Work out the finished part from the listing and answer in its coordinate system (mm). A direction names the side the tool comes from. Give positions to 0.01 mm unless a question says otherwise; leave off trailing zeros. Write each loop counter-clockwise with the first axis right and the second up, starting at its lowest first coordinate (ties: lowest second). Pieces come first, ordered by that corner, then holes. Notation, with made-up numbers: (-3, -9) - (35, -9) arc R20 ccw to (35, 23) - close; hole circle Ø10 at (32.25, 83). An arc over 180 degrees is marked (long way). Write item = value, one per line.
from build123d import *

# Parameters (mm, degrees)
SKETCH1_W                   = 190
SKETCH1_H                   = 175
SKETCH1_R                   = 2
SKETCH1_R_2                 = 1.75
BASE_DEPTH                  = 5.4
SKETCH3_R                   = 1.75
LONG_SIDE_CONNECTORS_DEPTH  = 5
SHORT_SIDE_CONNECTORS_DEPTH = 5
MIRROR3_COPY_1_DEPTH        = 5
CUT_EXTRUDE6_START          = -5.4
SKETCH11_R                  = 1.75
CUT_EXTRUDE6_DEPTH          = 179.761105811


with BuildPart() as part:
    # Sketch1 → Base (new body)
    with BuildSketch(Plane(origin=(0, 0, 0), x_dir=(1, 0, 0), z_dir=(0, 1, 0))):
        with Locations((-51.064381671, 5.614281477)):
            Rectangle(SKETCH1_W, SKETCH1_H)
        with Locations(Location((-26.064381671, 30.614281477, 0), (0, 0, 270))):
            Circle(SKETCH1_R, mode=Mode.SUBTRACT)
        with Locations(Location((-26.064381671, -19.385718523, 0), (0, 0, 270))):
            Circle(SKETCH1_R, mode=Mode.SUBTRACT)
        with Locations(Location((-26.064381671, -62.885718523, 0), (0, 0, 270))):
            Circle(SKETCH1_R_2, mode=Mode.SUBTRACT)
        with Locations(Location((-26.064381671, 74.114281477, 0), (0, 0, 270))):
            Circle(SKETCH1_R_2, mode=Mode.SUBTRACT)
        with Locations(Location((-93.064381671, 6.114281477, 0), (0, 0, 270))):
            Circle(SKETCH1_R_2, mode=Mode.SUBTRACT)
        with Locations(Location((-93.064381671, -63.885718523, 0), (0, 0, 270))):
            Circle(SKETCH1_R_2, mode=Mode.SUBTRACT)
    extrude(amount=-BASE_DEPTH)

    # Sketch3 → Long_Side_connectors (add)
    # profile 1 of 2: a face of its own
    with BuildSketch(Plane(origin=(-143.064381671, 0, 0), x_dir=(0, 0, -1), z_dir=(1, 0, 0))):
        with BuildLine():
            Line((76.114281477, 0), (90.114281477, 0))
            ThreePointArc((90.114281477, 0), (83.114281477, 7), (76.114281477, 0))
        make_face()
        with Locations((83.114281477, 4)):
            Circle(SKETCH3_R, mode=Mode.SUBTRACT)
    # profile 2 of 2: a face of its own
    with BuildSketch(Plane(origin=(-143.064381671, 0, 0), x_dir=(0, 0, -1), z_dir=(1, 0, 0))):
        with BuildLine():
            Line((-78.885718523, 0), (-64.885718523, 0))
            ThreePointArc((-64.885718523, 0), (-71.885718523, 7), (-78.885718523, 0))
        make_face()
        with Locations((-71.885718523, 4)):
            Circle(SKETCH3_R, mode=Mode.SUBTRACT)
    long_side_connectors = extrude(amount=LONG_SIDE_CONNECTORS_DEPTH)

    # Sketch4 → Short_side_connectors (add)
    with BuildSketch(Plane.XY.offset(78.885718523)):
        with BuildLine():
            ThreePointArc((-131.064381671, 7), (-136.014129139, 4.949747468), (-138.064381671, 0))
            Line((-138.064381671, 0), (-131.064381671, 0))
            Line((-131.064381671, 0), (-131.064381671, 2.25))
            ThreePointArc((-131.064381671, 2.25), (-132.814381671, 4), (-131.064381671, 5.75))
            Line((-131.064381671, 5.75), (-131.064381671, 7))
        make_face()
        with BuildLine():
            Line((-131.064381671, 2.25), (-131.064381671, 0))
            Line((-131.064381671, 0), (-124.064381671, 0))
            ThreePointArc((-124.064381671, 0), (-126.114634203, 4.949747468), (-131.064381671, 7))
            Line((-131.064381671, 7), (-131.064381671, 5.75))
            ThreePointArc((-131.064381671, 5.75), (-129.826944804, 5.237436867), (-129.314381671, 4))
            ThreePointArc((-129.314381671, 4), (-129.826944804, 2.762563133), (-131.064381671, 2.25))
        make_face()
        with BuildLine():
            ThreePointArc((-131.064381671, 7), (-136.014129139, 4.949747468), (-138.064381671, 0))
            Line((-138.064381671, 0), (-131.064381671, 0))
            Line((-131.064381671, 0), (-131.064381671, 2.25))
            ThreePointArc((-131.064381671, 2.25), (-132.814381671, 4), (-131.064381671, 5.75))
            Line((-131.064381671, 5.75), (-131.064381671, 7))
        make_face()
        with BuildLine():
            Line((-131.064381671, 2.25), (-131.064381671, 0))
            Line((-131.064381671, 0), (-124.064381671, 0))
            ThreePointArc((-124.064381671, 0), (-126.114634203, 4.949747468), (-131.064381671, 7))
            Line((-131.064381671, 7), (-131.064381671, 5.75))
            ThreePointArc((-131.064381671, 5.75), (-129.826944804, 5.237436867), (-129.314381671, 4))
            ThreePointArc((-129.314381671, 4), (-129.826944804, 2.762563133), (-131.064381671, 2.25))
        make_face()
    short_side_connectors = extrude(amount=-SHORT_SIDE_CONNECTORS_DEPTH)

    # Mirror1: Short_side_connectors across plane
    add(short_side_connectors.mirror(Plane.XY.offset(-5.614281477)))

    # Mirror3: Long_Side_connectors, Short_side_connectors across plane
    add(long_side_connectors.mirror(Plane(origin=(-51.064381671, 0, 0), x_dir=(0, 0, 1), z_dir=(1, 0, 0))))
    add(short_side_connectors.mirror(Plane(origin=(-51.064381671, 0, 0), x_dir=(0, 0, 1), z_dir=(1, 0, 0))))

    # Mirror3 copy 1 sketch → Mirror3 copy 1 (add)
    with BuildSketch(Plane(origin=(-102.128763342, 0, -90.114281477), x_dir=(-1, 0, 0), z_dir=(0, 0, -1))):
        with BuildLine():
            ThreePointArc((-131.064381671, 7), (-136.014129139, 4.949747468), (-138.064381671, 0))
            Line((-138.064381671, 0), (-131.064381671, 0))
            Line((-131.064381671, 0), (-131.064381671, 2.25))
            ThreePointArc((-131.064381671, 2.25), (-132.814381671, 4), (-131.064381671, 5.75))
            Line((-131.064381671, 5.75), (-131.064381671, 7))
        make_face()
        with BuildLine():
            Line((-131.064381671, 2.25), (-131.064381671, 0))
            Line((-131.064381671, 0), (-124.064381671, 0))
            ThreePointArc((-124.064381671, 0), (-126.114634203, 4.949747468), (-131.064381671, 7))
            Line((-131.064381671, 7), (-131.064381671, 5.75))
            ThreePointArc((-131.064381671, 5.75), (-129.826944804, 5.237436867), (-129.314381671, 4))
            ThreePointArc((-129.314381671, 4), (-129.826944804, 2.762563133), (-131.064381671, 2.25))
        make_face()
        with BuildLine():
            ThreePointArc((-131.064381671, 7), (-136.014129139, 4.949747468), (-138.064381671, 0))
            Line((-138.064381671, 0), (-131.064381671, 0))
            Line((-131.064381671, 0), (-131.064381671, 2.25))
            ThreePointArc((-131.064381671, 2.25), (-132.814381671, 4), (-131.064381671, 5.75))
            Line((-131.064381671, 5.75), (-131.064381671, 7))
        make_face()
        with BuildLine():
            Line((-131.064381671, 2.25), (-131.064381671, 0))
            Line((-131.064381671, 0), (-124.064381671, 0))
            ThreePointArc((-124.064381671, 0), (-126.114634203, 4.949747468), (-131.064381671, 7))
            Line((-131.064381671, 7), (-131.064381671, 5.75))
            ThreePointArc((-131.064381671, 5.75), (-129.826944804, 5.237436867), (-129.314381671, 4))
            ThreePointArc((-129.314381671, 4), (-129.826944804, 2.762563133), (-131.064381671, 2.25))
        make_face()
    extrude(amount=-MIRROR3_COPY_1_DEPTH)

    # Sketch11 → Cut-Extrude6 (cut, through all)
    with BuildSketch(Plane(origin=(0, 0, 0), x_dir=(1, 0, 0), z_dir=(0, 1, 0)).offset(CUT_EXTRUDE6_START)):
        with Locations(Location((-133.064381671, -63.885718523, 0), (0, 0, 90))):
            Circle(SKETCH11_R)
        with Locations(Location((-128.064381671, -68.885718523, 0), (0, 0, 90))):
            Circle(SKETCH11_R)
        with Locations(Location((-133.064381671, 75.114281477, 0), (0, 0, 90))):
            Circle(SKETCH11_R)
        with Locations(Location((-128.064381671, 80.114281477, 0), (0, 0, 90))):
            Circle(SKETCH11_R)
        with Locations(Location((30.935618329, -63.885718523, 0), (0, 0, 90))):
            Circle(SKETCH11_R)
        with Locations(Location((25.935618329, -68.885718523, 0), (0, 0, 90))):
            Circle(SKETCH11_R)
        with Locations(Location((30.935618329, 75.114281477, 0), (0, 0, 90))):
            Circle(SKETCH11_R)
        with Locations(Location((25.935618329, 80.114281477, 0), (0, 0, 90))):
            Circle(SKETCH11_R)
    extrude(amount=CUT_EXTRUDE6_DEPTH, mode=Mode.SUBTRACT)


solid = part.part
1. A tool of negligible diameter and unlimited length cuts with its end or side. For faces 1 (the cylindrical face through (38, 7, 72)), 2 (the flat face through (-131, 2, 73.886)), 3 (the flat face through (40.936, 2, 72)), 4 (the flat face through (29, 2, -90.114)), 5 (the cylindrical face through (-141, 7, 72)), from which of +Z, -Z, +X, -X, +Y, -Y can it reach the whole face along a straight path? Write none if from no direction.
Solution:
face_1 = +X, +Y
face_2 = +Y
face_3 = +Z, -Z, +X, +Y
face_4 = -Z, +X, -X, +Y
face_5 = -X, +Y
2. Find section B-B, the plane x = -7. Give the vertices of the cut face in (y, z), then the cut area to 3 significant figures.
Solution:
outline = (-5.4, -93.11) - (0, -93.11) - (0, 81.89) - (-5.4, 81.89) - close
area = 945 mm^2
3. Find section A-A, the plane z = 2.5. Give the vertices of the cut face in (x, y).
Solution:
outline = (-146.06, -5.4) - (43.94, -5.4) - (43.94, 0) - (-146.06, 0) - close
4. Given pin 1 (3 mm diameter, centred on y = 4, z = -83.11, fed in from -X); pin 2 (5.5 mm diameter, centred on x = -132, y = 3, fed in from -Z); pin 3 (6.5 mm diameter, centred on x = -26.06, z = 19.39, fed in from +Y); pin 4 (5.5 mm diameter, centred on x = -134.5, y = 3, fed in from +Z), each flat-ended and moving along its own axis, determine where each tip first touches the part or whether it passes through.
Solution:
pin_1 = through
pin_2 = -90.11
pin_3 = 0
pin_4 = 78.89
5. For a pull along Z with two mould halves and no side action, classify faces 6 (the flat face through (-131, 2, -90.114)), 7 (the flat face through (29, 2, 78.886)), 8 (the flat face through (43.936, -3, -4)), 9 (the flat face through (35.936, 2, 72)) as pulls with the +Z half, pulls with the -Z half, needs draft (parallel to the pull), parting line crosses it, or undercut.
Solution:
face_6 = pulls with the -Z half
face_7 = pulls with the +Z half
face_8 = needs draft
face_9 = undercut
6. Straight lines are drawn through the part: line 1 (Y direction, x = -58, z = 0.5); line 2 (Z direction, x = 26.5, y = 0.25); line 3 (X direction, y = -0.5, z = -74). For each, find the intervals that lie inside material, in ascending order.
Solution:
line_1 = -5.4 to 0
line_2 = -90.11 to -85.11, 73.89 to 78.89
line_3 = -146.06 to -134.41, -131.71 to -27.81, -24.32 to 29.59, 32.29 to 43.94
